Check sheet for the modelled part. Datum: model origin and axes. Units: mm. Round coordinates to 2 decimals unless told otherwise and drop trailing zeros. Loops run counter-clockwise (first coordinate to the right, second up) from the corner with the lowest first, then second, coordinate; pieces in that order, holes last. Notation, with made-up numbers: (-7.5, 75) - (7.5, 75) arc R32 cw to (7.5, 103) - close; hole circle Ø2 at (55, -0.5). An arc over 180 degrees is marked (long way). Return JSON: item names as keys, results as strings.
Autodesk Fusion 360 part; units mm, degrees
sketch "Sketch1" plane through (0, 0, 0) normal (1, 0, 0) x (0, 0, -1)
  line L0 (0, -270) -> (0, 0)
  dimension "d15" = 270
sketch "Sketch2" plane through (0, 0, 0) normal (0, 1, 0) x (1, 0, 0)
  line L0 (-6, 3) -> (-3, 3)
  line L1 (-3, 3) -> (-3, 2)
  line L2 (-3, 2) -> (-6, 2)
  line L3 (-6, 2) -> (-6, 3)
  dimension "d1" = 1
  dimension "d2" = 3
sweep "Sweep1" add profiles "Sketch2" path "Sketch1" along L0 section 1
sketch "Sketch3" plane through (0, 0, 0) normal (0, 0, 1) x (1, 0, 0)
  line L0 (-6.7324, 2.9105) -> (-2.2324, 2.9105)
  line L1 (-2.2324, 2.9105) -> (-2.2324, -0.0895)
  line L2 (-2.2324, -0.0895) -> (-6.7324, -0.0895)
  line L3 (-6.7324, -0.0895) -> (-6.7324, 2.9105)
  line L4 (-5.9523, 1.9141) -> (-2.9523, 1.9141)
  line L5 (-2.9523, 1.9141) -> (-2.9523, 0.9141)
  line L6 (-2.9523, 0.9141) -> (-5.9523, 0.9141)
  line L7 (-5.9523, 0.9141) -> (-5.9523, 1.9141)
  dimension "d9" = 3
  dimension "d10" = 1
  dimension "d11" = 3
  dimension "d12" = 4.5
extrude "Extrude1" add sketch "Sketch3" against normal blind 3
Q1. Scan lines: probe 1 along Y at (x, z) = (-3.7, -0.5); probe 2 along Z at (x, y) = (-4.1, -187.5); probe 3 along Y at (x, z) = (-4.3, -2.75). Record each from-to range of solid material in increasing order. Write a range as [from, to].
Answer key:
{"probe 1": "y = [-0.09, 0.91], [1.91, 2.91]", "probe 2": "z = [-3, -2]", "probe 3": "y = [-270, 0.91], [1.91, 2.91]"}
Q2. Sectioned sample at B-B (x = -5.2). Enter the section's corners in (y, z), plus the area to 3 significant figures.
Answer key:
{"outline": "(-270, -3) - (0.91, -3) - (0.91, 0) - (-0.09, 0) - (-0.09, -2) - (-270, -2) - close; (1.91, -3) - (2.91, -3) - (2.91, 0) - (1.91, 0) - close", "area": "276 mm²"}
Q3. Depth check by flat-ended pin: P1, Ø1.5, axis at x = -3, y = -79.5, coming from the +Z side; P2, Ø0.5, axis at y = -162, z = -2.5, coming from the -X side; P3, Ø1.1, axis at y = -111.5, z = -2.5, coming from the +X side. Enter the tip coordinate at first touch or a pass-through.
Answer key:
{"P1": "stops at z = -2", "P2": "stops at x = -6", "P3": "stops at x = -3"}
Q4. Sectioned sample at A-A (z = -0.45). Enter the section's corners in (x, y), plus the area to 3 significant figures.
Answer key:
{"outline": "(-6.73, -0.09) - (-2.23, -0.09) - (-2.23, 2.91) - (-6.73, 2.91) - close; hole (-5.95, 0.91) - (-2.95, 0.91) - (-2.95, 1.91) - (-5.95, 1.91) - close", "area": "10.5 mm²"}
Q5. Sectioned sample at C-C (y = -82.5). Enter the section's corners in (x, z).
Answer key:
{"outline": "(-6, -3) - (-3, -3) - (-3, -2) - (-6, -2) - close"}
